Model file for the job. Use its own axes, mm. Face numbers are marked on the shaded views. A direction names the side the tool comes from. Coordinates: 2 decimals unless noted, no trailing zeros. Write item = value, one per line. Start each with the question number.
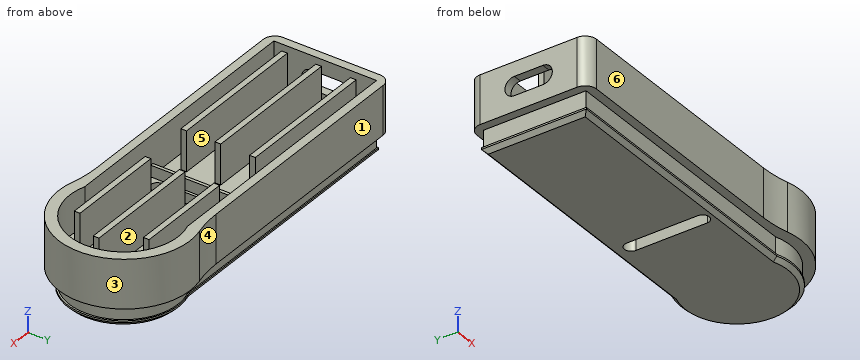
from build123d import *

# Parameters (mm, degrees)
PAD001_DEPTH    = 8.5
PAD002_DEPTH    = 3
FILLET008_R     = 20
FILLET009_R     = 20
FILLET010_R     = 2
FILLET011_R     = 2
POCKET002_DEPTH = 7
POCKET003_DEPTH = 5
PAD006_DEPTH    = 2
POCKET004_DEPTH = 5
PAD007_DEPTH    = 1
CHAMFER_SIZE    = 0.7
POCKET009_DEPTH = 5
SKETCH017_W     = 25
SKETCH017_H     = 1
SKETCH017_W_2   = 17.481396
SKETCH017_W_3   = 21.375297
SKETCH017_W_4   = 17.578514
PAD008_DEPTH    = 7


with BuildPart() as part:
    # Sketch004 → Pad001 (new body)
    with BuildSketch(Plane.XY.offset(80)):
        with BuildLine():
            Line((0.000991, 21), (46.615791, 21))
            ThreePointArc((46.615791, 0), (62.806207, 10.5), (46.615791, 21))
            Line((46.615791, 0), (0.000991, 0))
            Line((0.000991, 0), (0.000991, 21))
        make_face()
    extrude(amount=PAD001_DEPTH)

    # Sketch005 → Pad002 (new body)
    with BuildSketch(Plane(origin=(0, 0, 80), x_dir=(1, 0, 0), z_dir=(0, 0, -1))):
        with BuildLine():
            Line((1.502067, -19.500282), (48.477067, -19.500282))
            ThreePointArc((48.477067, -19.500282), (61.018448, -10.500282), (48.477067, -1.500282))
            Line((1.502067, -1.500282), (48.477067, -1.500282))
            Line((1.502067, -1.500282), (1.502067, -19.500282))
        make_face()
    extrude(amount=PAD002_DEPTH)

    # Fillet008
    fillet008_edges = [part.edges().sort_by_distance(p)[0] for p in [
        (46.615791, 21, 84.25),
    ]]
    fillet(fillet008_edges, radius=FILLET008_R)

    # Fillet009
    fillet009_edges = [part.edges().sort_by_distance(p)[0] for p in [
        (46.615791, 0, 84.25),
    ]]
    fillet(fillet009_edges, radius=FILLET009_R)

    # Fillet010
    fillet010_edges = [part.edges().sort_by_distance(p)[0] for p in [
        (0.000991, 0, 84.25),
    ]]
    fillet(fillet010_edges, radius=FILLET010_R)

    # Fillet011
    fillet011_edges = [part.edges().sort_by_distance(p)[0] for p in [
        (0.000991, 21, 84.25),
    ]]
    fillet(fillet011_edges, radius=FILLET011_R)

    # Sketch006 → Pocket002 (cut)
    with BuildSketch(Plane.XY.offset(88.5)):
        with BuildLine():
            Line((1.500423, 1.490874), (48.388216, 1.476974))
            ThreePointArc((48.388216, 1.476974), (60.908955, 10.483923), (48.388218, 19.490874))
            Line((1.500423, 19.490874), (48.388218, 19.490874))
            Line((1.500423, 19.490874), (1.500423, 1.490874))
        make_face()
    extrude(amount=-POCKET002_DEPTH, mode=Mode.SUBTRACT)

    # Sketch007 → Pocket003 (cut)
    with BuildSketch(Plane(origin=(0.000991, 0, 80), x_dir=(0, -1, 0), z_dir=(-1, 0, 0))):
        with BuildLine():
            ThreePointArc((-13.007468, 5.979853), (-14.65632, 4.331001), (-13.007468, 2.682149))
            Line((-13.007468, 2.682149), (-8.001338, 2.682149))
            ThreePointArc((-8.001338, 2.682149), (-6.352486, 4.331001), (-8.001338, 5.979853))
            Line((-13.007468, 5.979853), (-8.001338, 5.979853))
        make_face()
    extrude(amount=-POCKET003_DEPTH, mode=Mode.SUBTRACT)

    # Sketch012 → Pad006 (new body)
    with BuildSketch(Plane.XY.offset(81.5)):
        Polygon((31.498466, 19.496653), (31.498466, 1.452961), (32.048512, 1.452961), (32.059631, 19.496653), align=None)
    extrude(amount=PAD006_DEPTH)

    # Sketch013 → Pocket004 (cut)
    with BuildSketch(Plane.XY.offset(81.5)):
        with BuildLine():
            ThreePointArc((34.843688, 16.341736), (33.680227, 17.505197), (32.516766, 16.341736))
            Line((32.516766, 16.341736), (32.516766, 3.815891))
            ThreePointArc((32.516766, 3.815891), (33.680227, 2.65243), (34.843688, 3.815891))
            Line((34.843688, 16.341736), (34.843688, 3.815891))
        make_face()
    extrude(amount=-POCKET004_DEPTH, mode=Mode.SUBTRACT)

    # Sketch015 → Pad007 (new body)
    with BuildSketch(Plane(origin=(0, 0, 77), x_dir=(1, 0, 0), z_dir=(0, 0, -1))):
        with BuildLine():
            Line((1.311159, -1.309228), (48.561159, -1.309228))
            ThreePointArc((48.561159, -19.709228), (61.335244, -10.509228), (48.561159, -1.309228))
            Line((48.561159, -19.709228), (1.311159, -19.709228))
            Line((1.311159, -19.709228), (1.311159, -1.309228))
        make_face()
    extrude(amount=PAD007_DEPTH)

    # Chamfer
    chamfer_edges = [part.edges().sort_by_distance(p)[0] for p in [
        (1.311159, 10.509228, 76),
        (24.936159, 1.309228, 76),
        (24.936159, 19.709228, 76),
        (61.335244, 10.509228, 76),
    ]]
    chamfer(chamfer_edges, length=CHAMFER_SIZE)

    # Sketch016 → Pocket009 (cut)
    with BuildSketch(Plane.XY.offset(77)):
        with BuildLine():
            ThreePointArc((34.843688, 16.341736), (33.680227, 17.505197), (32.516766, 16.341736))
            Line((32.516766, 16.341736), (32.516766, 3.815891))
            ThreePointArc((32.516766, 3.815891), (33.680227, 2.65243), (34.843688, 3.815891))
            Line((34.843688, 16.341736), (34.843688, 3.815891))
        make_face()
    extrude(amount=-POCKET009_DEPTH, mode=Mode.SUBTRACT)

    # Sketch017 → Pad008 (new body)
    with BuildSketch(Plane.XY.offset(81.5)):
        with Locations((15.546838, 16.499521)):
            Rectangle(SKETCH017_W, SKETCH017_H)
        with Locations((15.512423, 10.408272)):
            Rectangle(SKETCH017_W, SKETCH017_H)
        with Locations((15.512423, 4.420265)):
            Rectangle(SKETCH017_W, SKETCH017_H)
        with Locations((45.692045, 16.535934)):
            Rectangle(SKETCH017_W_2, SKETCH017_H)
        with Locations((47.570167, 10.442687)):
            Rectangle(SKETCH017_W_3, SKETCH017_H)
        with Locations((45.706188, 4.454679)):
            Rectangle(SKETCH017_W_4, SKETCH017_H)
    extrude(amount=PAD008_DEPTH)


solid = part.part
Item 1: 3-axis set-ups, long thin cutter, end or side, ignore diameter. For the marked faces 1, 2 and 3: which of +Z, -Z, +X, -X, +Y, -Y reach the whole face in a straight line?
Item 2: Cut at B-B (y = 11.5). Give the number of separate pieces and of enclosed holes in the cut face, plus the area to 3 significant figures.
Item 3: Pin check, flat tips, straight feed: pin 1 Ø3 at (x, y) = (33.5, 13) entering from +Z; pin 2 Ø0.5 at (y, z) = (16.5, 84.5) entering from +X; pin 3 Ø2 at (x, z) = (24.5, 83.5) entering from +Y. Stop position of each tip, or through.
Item 4: Pull direction X, two halves, no side cores. Call the marked faces 4, 5 and 6: +X half, -X half, draft (parallel to the pull), parting line (faces both ways), or undercut.
Item 5: Probe L1, parallel to Y at x = 20.5, z = 84; L2, parallel to Y at x = 57.5, z = 87.75; L3, parallel to Y at x = 48, z = 82.5. List the from-to ranges inside material, lowest first.
Reported:
q1.face_1 = +Z, -Z, -X, +Y
q1.face_2 = +Z
q1.face_3 = +Z, -Z
q2.separate_pieces = 3
q2.enclosed_holes = 0
q2.area = 339 mm^2
q3.pin_1 = 83.5
q3.pin_2 = 61.27
q3.pin_3 = 21
q4.face_4 = -X half
q4.face_5 = undercut
q4.face_6 = draft
q5.L1 = 0 to 1.49, 3.92 to 4.92, 9.91 to 10.91, 16 to 17, 19.49 to 21
q5.L2 = 0.81 to 3.19, 9.94 to 10.94, 17.77 to 20.19
q5.L3 = -0.53 to 1.48, 3.95 to 4.95, 9.94 to 10.94, 16.04 to 17.04, 19.49 to 21.53
